Read the model definition and answer for the solid it produces. Units are mm, in the model's axes. A direction names the side the tool comes from. Round coordinates to 2 decimals unless told otherwise and drop trailing zeros. Loops run counter-clockwise (first coordinate to the right, second up) from the corner with the lowest first, then second, coordinate; pieces in that order, holes last. Notation, with made-up numbers: M 85.25,34 L 109.25,34 A21 cw 109.25,58 Z; hole C -34,1 d7. An arc over 180 degrees is marked long. Answer as CSV lines item,"result".
```python
from build123d import *

# Parameters (mm, degrees)
SKETCH1_R                  = 1.7500000000000038
SKETCH1_R_2                = 1.7500000000000033
BASE_FLANGE1_DEPTH         = 2
SKETCHED_START             = -55
SKETCHED_BEND1_DEPTH       = 14
SKETCHED_START_2           = -48.2499999
SKETCHED_BEND1_2_DEPTH     = 7.2499999
SKETCHED_BEND1_3_DEPTH     = 3.2499999
SKETCHED_START_3           = -51.7500001
SKETCHED_BEND1_4_DEPTH     = 3.5000002
SKETCHED_START_4           = -10.9966
SKETCHED_BEND1_5_OUTLINE_R = 1.75
SKETCHED_BEND1_5_DEPTH     = 19.0032
FILLET1_R                  = 5
CUT_EXTRUDE2_REACH         = 70.738
FILLET2_R                  = 5
BOSS_EXTRUDE1_START        = 2
SKETCH9_R                  = 1.7500000000000036
BOSS_EXTRUDE1_DEPTH        = 2
CUT_EXTRUDE1_REACH         = 72.286
SKETCH7_R                  = 0.24999999999999958
SKETCH10_R                 = 1.7500000000000036
BOSS_EXTRUDE2_DEPTH        = 2
FILLET3_R                  = 2


with BuildPart() as part:
    # Base-Flange1: sheet metal written as solids
    # Sketch1 → Base-Flange1 (new body)
    with BuildSketch(Plane.XY):
        with BuildLine():
            Line((-39.65131901967449, 5.269999999999999), (-40.999999999999986, 5.270000000000006))
            Line((-40.999999999999986, 5.270000000000006), (-40.999999999999986, 17.26000000000001))
            Line((-40.999999999999986, 17.26000000000001), (-54.999999999999986, 17.260000000000012))
            Line((-54.999999999999986, 17.260000000000012), (-54.99999999999998, -20.25))
            Line((-54.99999999999998, -20.25), (-40.99999999999998, -20.250000000000004))
            Line((-40.99999999999998, -20.250000000000004), (-40.999999999999986, -8.26))
            Line((-40.999999999999986, -8.26), (-39.13786401938665, -8.26))
            ThreePointArc((-39.13786401938665, -8.26), (-9.571278660785763, -38.83800490238379), (30.81801421246995, -25.500000000000004))
            Line((30.81801421246995, -25.500000000000004), (43, -25.5))
            Line((43, -25.5), (43, -15.499999999999998))
            Line((43, -15.499999999999998), (36.874788134984584, -15.499999999999996))
            ThreePointArc((36.874788134984584, -15.499999999999996), (10.47738068118216, 38.60342593684647), (-39.65131901967449, 5.269999999999999))
        make_face()
        with Locations((-50, 12.260000000000014)):
            Circle(SKETCH1_R, mode=Mode.SUBTRACT)
        with Locations(Location((-49.999999999999986, -15.250000000000002, 0), (0, 0, 180))):
            Circle(SKETCH1_R_2, mode=Mode.SUBTRACT)
    extrude(amount=-BASE_FLANGE1_DEPTH)

    # Sketched Bend1: read off the stored shape, not the designer's step
    # Sketched Bend1 outline → Sketched Bend1 (cut)
    with BuildSketch(Plane.YZ.offset(SKETCHED_START)):
        with BuildLine():
            Line((-20.25, -2), (-8.26, -2))
            ThreePointArc((-8.26, -2), (-9.914267209, -1.443395312), (-10.895602398, 0))
            Line((-10.895602398, 0), (-20.25, 0))
            Line((-20.25, 0), (-20.25, -2))
        make_face()
        with BuildLine():
            ThreePointArc((7.905602398, 0), (6.924267209, -1.443395312), (5.27, -2))
            Line((5.27, -2), (17.26, -2))
            Line((17.26, -2), (17.26, 0))
            Line((17.26, 0), (7.905602398, 0))
        make_face()
    extrude(amount=SKETCHED_BEND1_DEPTH, mode=Mode.SUBTRACT)

    # Sketched Bend1 2 outline → Sketched Bend1 2 (add)
    with BuildSketch(Plane.YZ.offset(SKETCHED_START_2)):
        with BuildLine():
            ThreePointArc((-10.9966, 0.7366), (-10.971233029, 0.364854094), (-10.895602398, 0))
            Line((-10.895602398, 0), (-8.26, 0))
            ThreePointArc((-8.26, 0), (-8.780854855, 0.215745145), (-8.9966, 0.7366))
            Line((-8.9966, 0.7366), (-8.9966, 9.998755099))
            Line((-8.9966, 9.998755099), (-10.9966, 9.998755099))
            Line((-10.9966, 9.998755099), (-10.9966, 0.7366))
        make_face()
        with BuildLine():
            Line((5.27, 0), (7.905602398, 0))
            ThreePointArc((7.905602398, 0), (7.981233029, 0.364854094), (8.0066, 0.7366))
            Line((8.0066, 0.7366), (8.0066, 9.998755099))
            Line((8.0066, 9.998755099), (6.0066, 9.998755099))
            Line((6.0066, 9.998755099), (6.0066, 0.7366))
            ThreePointArc((6.0066, 0.7366), (5.790854855, 0.215745145), (5.27, 0))
        make_face()
    extrude(amount=SKETCHED_BEND1_2_DEPTH)

    # Sketched Bend1 3 outline → Sketched Bend1 3 (add)
    with BuildSketch(Plane.YZ.offset(SKETCHED_START)):
        with BuildLine():
            ThreePointArc((-10.9966, 0.7366), (-10.971233029, 0.364854094), (-10.895602398, 0))
            Line((-10.895602398, 0), (-8.26, 0))
            ThreePointArc((-8.26, 0), (-8.780854855, 0.215745145), (-8.9966, 0.7366))
            Line((-8.9966, 0.7366), (-8.9966, 9.998755099))
            Line((-8.9966, 9.998755099), (-10.9966, 9.998755099))
            Line((-10.9966, 9.998755099), (-10.9966, 0.7366))
        make_face()
        with BuildLine():
            Line((5.27, 0), (7.905602398, 0))
            ThreePointArc((7.905602398, 0), (7.981233029, 0.364854094), (8.0066, 0.7366))
            Line((8.0066, 0.7366), (8.0066, 9.998755099))
            Line((8.0066, 9.998755099), (6.0066, 9.998755099))
            Line((6.0066, 9.998755099), (6.0066, 0.7366))
            ThreePointArc((6.0066, 0.7366), (5.790854855, 0.215745145), (5.27, 0))
        make_face()
    extrude(amount=SKETCHED_BEND1_3_DEPTH)

    # Sketched Bend1 4 outline → Sketched Bend1 4 (add)
    with BuildSketch(Plane.YZ.offset(SKETCHED_START_3)):
        with BuildLine():
            ThreePointArc((6.0066, 0.7366), (5.790854855, 0.215745145), (5.27, 0))
            Line((5.27, 0), (7.905602398, 0))
            ThreePointArc((7.905602398, 0), (7.981233029, 0.364854094), (8.0066, 0.7366))
            Line((8.0066, 0.7366), (8.0066, 9.998755099))
            Line((8.0066, 9.998755099), (6.0066, 9.998755099))
            Line((6.0066, 9.998755099), (6.0066, 0.7366))
        make_face()
        with BuildLine():
            ThreePointArc((-10.9966, 0.7366), (-10.971233029, 0.364854094), (-10.895602398, 0))
            Line((-10.895602398, 0), (-8.26, 0))
            ThreePointArc((-8.26, 0), (-8.780854855, 0.215745145), (-8.9966, 0.7366))
            Line((-8.9966, 0.7366), (-8.9966, 9.998755099))
            Line((-8.9966, 9.998755099), (-10.9966, 9.998755099))
            Line((-10.9966, 9.998755099), (-10.9966, 0.7366))
        make_face()
    extrude(amount=SKETCHED_BEND1_4_DEPTH)

    # Sketched Bend1 5 outline → Sketched Bend1 5 (cut)
    with BuildSketch(Plane(origin=(0, 0, 0), x_dir=(1, 0, 0), z_dir=(0, 1, 0)).offset(SKETCHED_START_4)):
        with Locations((-50, -4.998755099)):
            Circle(SKETCHED_BEND1_5_OUTLINE_R)
    extrude(amount=SKETCHED_BEND1_5_DEPTH, mode=Mode.SUBTRACT)

    # Fillet1
    # the kernel refuses this fillet: 5 mm, written as the material it adds along each edge
    with BuildSketch(Plane(origin=(30.818014212469954, -25.500000000000007, 0), x_dir=(-0.6578741358493351, -0.7531278917823256, 0), z_dir=(0, 0, -1))) as fillet1_piece_1:
        with BuildLine():
            CenterArc((2.272928109865178, -4.998212067114161), FILLET1_R, 91.53229073869478, 47.329766128742406)
            Line((-1.49271134904645, -1.7088413878674857), (-1.5680241382246838, -1.6430539742825514))
            Line((-1.5680241382246838, -1.6430539742825514), (-0.07531278917823364, 0.06578741358493444))
            Line((-0.07531278917823364, 0.06578741358493444), (0.00267403307043032, 0.09996424134228217))
            ThreePointArc((0.00267403307043032, 0.09996424134228217), (1.0696132281718547, 0.0856965369132901), (2.1365524232732724, 0.0999642413422845))
            Line((2.1365524232732724, 0.0999642413422845), (2.139226456343701, -1e-16))
        make_face()
    extrude(amount=2)
    with BuildSketch(Plane(origin=(36.874788134984584, -15.499999999999996, 0), x_dir=(0.3120481831654017, 0.9500662773634121, 0), z_dir=(0, 0, -1))) as fillet1_piece_2:
        with BuildLine():
            CenterArc((6.841047896129056, 4.983779941379127), FILLET1_R, 170.3798521279212, 95.00382355421686)
            Line((1.911361233981272, 5.8193572346573905), (1.8127675007383173, 5.836068780522958))
            ThreePointArc((1.8127675007383173, 5.836068780522958), (0.8606739892542704, 2.9408834356452394), (-0.09500662773634087, 0.03120481831654006))
            Line((-0.09500662773634087, 0.03120481831654006), (0.00804829164250585, -0.09967559882757966))
            ThreePointArc((0.00804829164250585, -0.09967559882757966), (3.219316657001906, 0.02976046896695109), (6.430585022361307, -0.09967559882758435))
            Line((6.430585022361307, -0.09967559882758435), (6.438633314003813, 2.9e-16))
        make_face()
    extrude(amount=2)

    # Sketch8 → Cut-Extrude2 (cut, up to next)
    with BuildSketch(Plane.XY, mode=Mode.PRIVATE) as cut_extrude2_sk1:
        with BuildLine():
            Line((10.500000000000004, -38.59727969689056), (10.50000000000001, -36))
            ThreePointArc((10.500000000000012, -36), (4.4e-16, -37.5), (-10.50000000000001, -36))
            Line((-10.50000000000001, -36), (-10.499999999999996, -38.59727969689056))
            ThreePointArc((-10.499999999999998, -38.59727969689057), (2.22e-15, -40.00000000000001), (10.499999999999998, -38.59727969689057))
        make_face()
    cut_extrude2_tool1 = extrude(cut_extrude2_sk1.sketch, amount=-CUT_EXTRUDE2_REACH, mode=Mode.PRIVATE) & part.part
    # Sketch8 → Cut-Extrude2 (cut, up to next)
    with BuildSketch(Plane.XY, mode=Mode.PRIVATE) as cut_extrude2_sk2:
        with BuildLine():
            ThreePointArc((10.5, 35.99999999999999), (2.3e-15, 37.49999999999999), (-10.5, 35.99999999999999))
            Line((-10.5, 35.99999999999999), (-10.500000000000004, 38.59727969689055))
            ThreePointArc((-10.500000000000004, 38.59727969689055), (2.45e-15, 39.99999999999999), (10.499999999999996, 38.59727969689055))
            Line((10.499999999999996, 38.59727969689055), (10.5, 35.99999999999999))
        make_face()
    cut_extrude2_tool2 = extrude(cut_extrude2_sk2.sketch, amount=-CUT_EXTRUDE2_REACH, mode=Mode.PRIVATE) & part.part
    add(cut_extrude2_tool1.solids().sort_by_distance((0, -38.265011, 0))[0], mode=Mode.SUBTRACT)
    add(cut_extrude2_tool2.solids().sort_by_distance((0, 38.265011, 0))[0], mode=Mode.SUBTRACT)

    # Fillet2
    fillet2_edges = [part.edges().sort_by_distance(p)[0] for p in [
        (-55, 7.006600000000001, 9.998755099),
        (-41, 7.006600000000001, 9.998755099),
        (-41, -9.9966, 9.998755099),
        (-55, -9.9966, 9.998755099),
    ]]
    fillet(fillet2_edges, radius=FILLET2_R)

    # Sketch9 → Boss-Extrude1 (add)
    with BuildSketch(Plane.XZ.offset(-6.006600000000028).offset(BOSS_EXTRUDE1_START)):
        with BuildLine():
            Line((-54.999999999999986, 0.7365999999999726), (-54.999999999999986, -1.843e-14))
            Line((-54.999999999999986, -1.843e-14), (-40.999999999999986, -1.843e-14))
            Line((-40.999999999999986, -1.843e-14), (-40.999999999999986, 0.7365999999999743))
            Line((-40.999999999999986, 0.7365999999999743), (-40.999999999999986, 4.998755098887944))
            ThreePointArc((-40.999999999999986, 4.998755098887944), (-42.46446609406725, 8.534289004820682), (-45.999999999999986, 9.998755098887946))
            Line((-45.999999999999986, 9.998755098887946), (-49.999999999999986, 9.998755098887948))
            ThreePointArc((-49.999999999999986, 9.998755098887948), (-53.53553390593273, 8.53428900482069), (-54.999999999999986, 4.99875509888795))
            Line((-54.999999999999986, 4.99875509888795), (-54.999999999999986, 0.7365999999999726))
        make_face()
        with Locations(Location((-50, 4.998755098887954, 0), (0, 0, 180))):
            Circle(SKETCH9_R, mode=Mode.SUBTRACT)
    extrude(amount=-BOSS_EXTRUDE1_DEPTH)

    # Sketch7 → Cut-Extrude1 (cut, up to next)
    with BuildSketch(Plane.XZ.offset(-4.006600000000027), mode=Mode.PRIVATE) as cut_extrude1_sk1:
        with Locations(Location((-44.00000000000001, 2.998755098887952, 0), (0, 0, 270))):
            Circle(SKETCH7_R)
    cut_extrude1_tool1 = extrude(cut_extrude1_sk1.sketch, amount=-CUT_EXTRUDE1_REACH, mode=Mode.PRIVATE) & part.part
    add(cut_extrude1_tool1.solids().sort_by_distance((-44, 4.0066, 2.998755))[0], mode=Mode.SUBTRACT)

    # Sketch10 → Boss-Extrude2 (add)
    with BuildSketch(Plane(origin=(0, -8.996599999999987, 3.141e-14), x_dir=(1, 0, 0), z_dir=(0, 1, -3.49e-15))):
        with BuildLine():
            Line((-54.99999999999998, 2.884e-14), (-54.99999999999998, -0.7365999999999777))
            Line((-54.99999999999998, -0.7365999999999777), (-54.99999999999998, -4.99875509888795))
            ThreePointArc((-54.99999999999998, -4.99875509888795), (-53.535533905932716, -8.534289004820696), (-49.99999999999997, -9.998755098887964))
            Line((-49.99999999999997, -9.998755098887964), (-45.99999999999998, -9.998755098887965))
            ThreePointArc((-45.99999999999998, -9.998755098887965), (-42.46446609406724, -8.534289004820701), (-40.99999999999998, -4.998755098887962))
            Line((-40.99999999999998, -4.998755098887962), (-40.999999999999986, -0.7365999999999864))
            Line((-40.999999999999986, -0.7365999999999864), (-40.999999999999986, 2.884e-14))
            Line((-40.999999999999986, 2.884e-14), (-54.99999999999998, 2.884e-14))
        make_face()
        with Locations(Location((-49.999999999999986, -4.9987550988879645, 0), (0, 0, 270))):
            Circle(SKETCH10_R, mode=Mode.SUBTRACT)
    extrude(amount=BOSS_EXTRUDE2_DEPTH)

    # Fillet3
    fillet3_edges = [part.edges().sort_by_distance(p)[0] for p in [
        (-47.999999999999986, 4.006600000000022, -4.44e-15),
        (-47.999999999999986, -6.996599999999987, -4.41e-15),
    ]]
    fillet(fillet3_edges, radius=FILLET3_R)


solid = part.part
```
1) Each of these flat-tipped pins is pushed along its axis until it touches: P1, Ø0.6, axis at x = -40, z = -0.5, coming from the -Y side; P2, Ø2.5, axis at x = -46, z = 4.5, coming from the +Y side; P3, Ø1, axis at y = -37.5, z = -1.5, coming from the -X side. Where does it stop, or does it pass through?
Evaluation:
P1,"stops at y = -8.26"
P2,"stops at y = 8.01"
P3,"stops at x = -15.2"
2) Straight lines are drawn through the part: line 1 (Z direction, x = -50, y = 5.45); line 2 (X direction, y = 5.5, z = 4.75); line 3 (Z direction, x = 5, y = -22). For each, find the intervals that lie inside material, in ascending order.
Evaluation:
line 1,"z = -1.99 to 3.25, 6.75 to 10"
line 2,"x = -55 to -51.73, -48.27 to -41"
line 3,"z = -2 to 0"
3) Find section A-A, the plane x = 9. Give the vertices of the cut face in (y, z), then the cut area to 3 significant figures.
Evaluation:
outline,"M -36.4,-2 L 36.4,-2 L 36.4,0 L -36.4,0 Z"
area,"146 mm^2"
4) A tool of negligible diameter and unlimited length cuts with its end or side. For faces 1 (the flat face through (10.5, -37, -1)), 2 (the flat face through (-41, 6, 2)), 3 (the cylindrical face through (-48.098, -6.395, 0.57)), 4 (the cylindrical face through (-48.098, -10.216, -1.177)), 5 (the flat face through (10.5, 37, -1)), from which of +Z, -Z, +X, -X, +Y, -Y can it reach the whole face along a straight path? Write none if from no direction.
Evaluation:
face 1,"+Z, -Z, -Y"
face 2,"+Z, +Y"
face 3,"+Z, +X, -X"
face 4,"-Z, -X, -Y"
face 5,"+Z, -Z, +Y"
5) Determine the mould class of faces 6 (the flat face through (-48, 8.007, 5)), 7 (the cylindrical face through (-43, 6, 9)), 8 (the flat face through (-48, 4.007, 6)) for opening direction Y: released by +Y, released by -Y, zero draft, split by the parting line, or undercut.
Evaluation:
face 6,"released by +Y"
face 7,"zero draft"
face 8,"undercut"
6) Find section B-B, the plane y = 29. Give the vertices of the cut face in (x, z), then the cut area to 3 significant figures.
Evaluation:
outline,"M -27.55,-2 L 27.55,-2 L 27.55,0 L -27.55,0 Z"
area,"110 mm^2"
